Check sheet for the drawn part. Datum: minimum x, y, z corner. Units: mm. A direction names the side the tool comes from. Round coordinates to 2 decimals unless told otherwise and drop trailing zeros. Write each loop counter-clockwise with the first axis right and the second up, starting at its lowest first coordinate (ties: lowest second). Pieces come first, ordered by that corner, then holes. Notation, with made-up numbers: (45.25, -12.75) - (78.25, -12.75) arc R21 cw to (78.25, 0.25) - close; hole circle Ø2 at (21.25, 51). An arc over 180 degrees is marked (long way). Write each question's results on one line, items separated by ' | '.
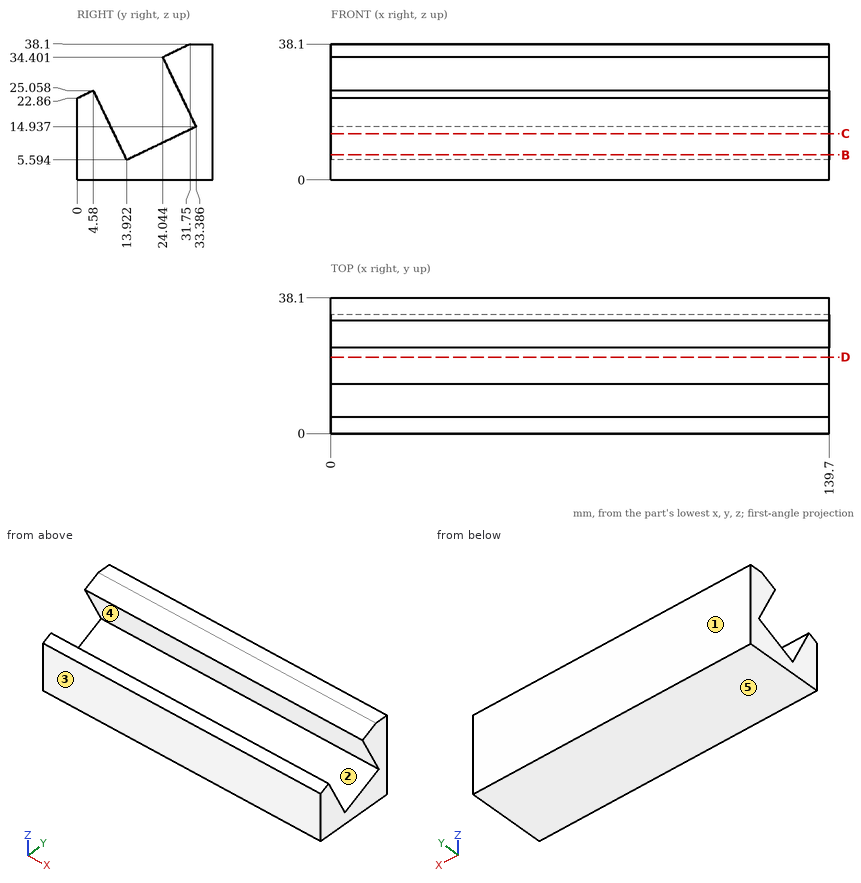
(1) Mould release check, pull along Z, two halves, no side actions. Record for the marked faces 3, 4 and 5: released by +Z, released by -Z, zero draft, split by the parting line, or undercut.
Answer:
face 3: zero draft | face 4: undercut | face 5: released by -Z
(2) Go/stop test with a flat-tipped pin: pin 1 Ø1.5 at (x, z) = (112, 14.5) entering from -Y. Record where the tip stops, or that it passes through.
Answer:
pin 1: y = 0
(3) Thickness scan on L1, parallel to Y at x = 38, z = 8 (1 decimal); L2, parallel to Y at x = 6.5, z = 10.5 (1 decimal); L3, parallel to Z at x = 74.5, y = 28.5 (1 decimal). Record the ranges inside material, lowest first.
Answer:
L1: 0 to 12.8, 18.9 to 38.1 | L2: 0 to 11.6, 24.1 to 38.1 | L3: 0 to 12.6, 25.1 to 36.5
(4) Set-up check for the marked faces 1 and 2: record each of +Z, -Z, +X, -X, +Y, -Y from which the full face is reachable in a straight line by a thin tool's end or side.
Answer:
face 1: +Z, -Z, +X, -X, +Y | face 2: +X, -X
(5) Section check C-C (z = 13). Record the cut outline in (x, y).
Answer:
outline: (0, 0) - (139.7, 0) - (139.7, 10.37) - (0, 10.37) - close; (0, 29.35) - (139.7, 29.35) - (139.7, 38.1) - (0, 38.1) - close
(6) Section check B-B (z = 7). Record the cut outline in (x, y), plus the area to 3 significant figures.
Answer:
outline: (0, 0) - (139.7, 0) - (139.7, 13.25) - (0, 13.25) - close; (0, 16.85) - (139.7, 16.85) - (139.7, 38.1) - (0, 38.1) - close | area: 4,820 mm2
(7) Section check D-D (y = 21.5). Record the cut outline in (x, z), plus the area to 3 significant figures.
Answer:
outline: (0, 0) - (139.7, 0) - (139.7, 9.23) - (0, 9.23) - close | area: 1,290 mm2
